```python
from build123d import *

# Parameters (mm, degrees)
F0_W        = 127
F0_H        = 76.2
F0_R        = 6.35
F1_DEPTH    = 50.8
F2_R        = 9.1340050973
F3_DEPTH    = 70.104
F4_T1_DEPTH = 192.3207478943
F5_R        = 12.7


# Not quite as in the source:
# - a fillet or chamfer that OpenCascade refuses, or shapes differently, is made with other operations: its cross-section is extruded or revolved along the edge and cut away or added


with BuildPart() as f1:
    # F0 (on Front) → F1 (new body)
    with BuildSketch(Plane.XZ):
        with Locations((4.9776248634, -39.8979571181)):
            Rectangle(F0_W, F0_H)
        with Locations((-33.1223751366, -27.1979571181)):
            Circle(F0_R, mode=Mode.SUBTRACT)
        with Locations((49.4276248634, -27.1979571181)):
            Circle(F0_R, mode=Mode.SUBTRACT)
    extrude(amount=F1_DEPTH)

    # F2 (on face) → F3 (cut)
    with BuildSketch(Plane.XZ.offset(50.8)):
        with Locations((-3.571436042, -21.4178189635)):
            Circle(F2_R)
    extrude(amount=-F3_DEPTH, mode=Mode.SUBTRACT)

    # F4: chamfer of 12.7 on 1 edges, made by hand

    # F4_s2 → F4_t1 (cut)
    with BuildSketch(Plane.YZ.offset(-91.1827490838)):
        Polygon((-38.1, -1.7979571181), (-50.8, -14.4979571181), (-50.8, -1.7979571181), align=None)
    extrude(amount=F4_T1_DEPTH, mode=Mode.SUBTRACT)

    # F5
    f5_edges = [f1.edges().sort_by_distance(p)[0] for p in [
        (-58.522375, -19.05, -1.797957),
    ]]
    fillet(f5_edges, radius=F5_R)


solid = f1.part
```
Check sheet for the modelled part. Datum: model origin and axes. Units: mm. Round coordinates to 2 decimals unless told otherwise and drop trailing zeros. Loops run counter-clockwise (first coordinate to the right, second up) from the corner with the lowest first, then second, coordinate; pieces in that order, holes last. Notation, with made-up numbers: (88, 62) -> (131, 62) arc R23 ccw to (131, 89) -> close; hole circle Ø3 at (-22, -16.75). An arc over 180 degrees is marked (long way). Write item = value, one per line. Start each with the question number.
1) Release check for a two-part mould opening along X. For faces 1 (the flat face through (-58.522, -25, -47)), 2 (the flat face through (4, -50.8, -46)), 3 (the cylindrical face through (-33.949, -25.044, -20.902)) record: released by +X, released by -X, zero draft, split by the parting line, or undercut.
2) Sectioned sample at B-B, the plane z = -23. Record the cut outline in (x, y), plus the area to 3 significant figures.
3) Gauge pin test, flat end, axial feed: pin 1 Ø16.5 at (x, z) = (-3.57, -21.42) entering from +Y. Record the tip position at first contact, or that the pin passes through.
4) Sectioned sample at D-D, the plane x = 4. Record the cut outline in (y, z), plus the area to 3 significant figures.
5) Sectioned sample at A-A, the plane y = -14. Record the cut outline in (x, z).
6) Thickness scan on probe 1 along Z at (x, y) = (49.5, -35); probe 2 along Z at (x, y) = (53, -35); probe 3 along X at (y, z) = (-25, -25). Record the ranges inside material, lowest first.
7) Sectioned sample at C-C, the plane x = 18.5. Record the cut outline in (y, z).
Results are:
q1.face_1 = released by -X
q1.face_2 = zero draft
q1.face_3 = undercut
q2.outline = (-58.52, -50.8) -> (-37.89, -50.8) -> (-37.89, 0) -> (-58.52, 0) -> close; (-28.36, -50.8) -> (-12.57, -50.8) -> (-12.57, 0) -> (-28.36, 0) -> close; (5.42, -50.8) -> (44.66, -50.8) -> (44.66, 0) -> (5.42, 0) -> close; (54.19, -50.8) -> (68.48, -50.8) -> (68.48, 0) -> (54.19, 0) -> close
q2.area = 4,570 mm^2
q3.pin_1 = through
q4.outline = (-50.8, -78) -> (0, -78) -> (0, -26.53) -> (-50.8, -26.53) -> close; (-50.8, -16.31) -> (0, -16.31) -> (0, -1.8) -> (-38.1, -1.8) -> (-50.8, -14.5) -> close
q4.area = 3,270 mm^2
q5.outline = (-58.52, -78) -> (68.48, -78) -> (68.48, -1.8) -> (-45.82, -1.8) arc R12.7 ccw to (-58.52, -14.5) -> close; hole circle Ø12.7 at (-33.12, -27.2); hole circle Ø18.27 at (-3.57, -21.42); hole circle Ø12.7 at (49.43, -27.2)
q6.probe_1 = -78 to -33.55, -20.85 to -1.8
q6.probe_2 = -78 to -32.45, -21.95 to -1.8
q6.probe_3 = -58.52 to -39.08, -27.16 to -11.97, 4.83 to 43.47, 55.39 to 68.48
q7.outline = (-50.8, -78) -> (0, -78) -> (0, -1.8) -> (-38.1, -1.8) -> (-50.8, -14.5) -> close
